Answer from the drawing. Dimensions are ordinates in mm from the lowest x, y and z of the part. A direction names the side the tool comes from. Coordinates: 2 decimals unless noted, no trailing zeros. Order: outer loops, then holes, each group sorted by start corner. A loop starts at its lowest first (then second) coordinate and runs counter-clockwise, first axis right, second up. Notation, with made-up numbers: (11, -3.75) -> (20, -3.75) arc R12 ccw to (20, 17.25) -> close; hole circle Ø2 at (52, -4.5). An arc over 180 degrees is marked (long way). Answer in a Markdown table with one row per item.
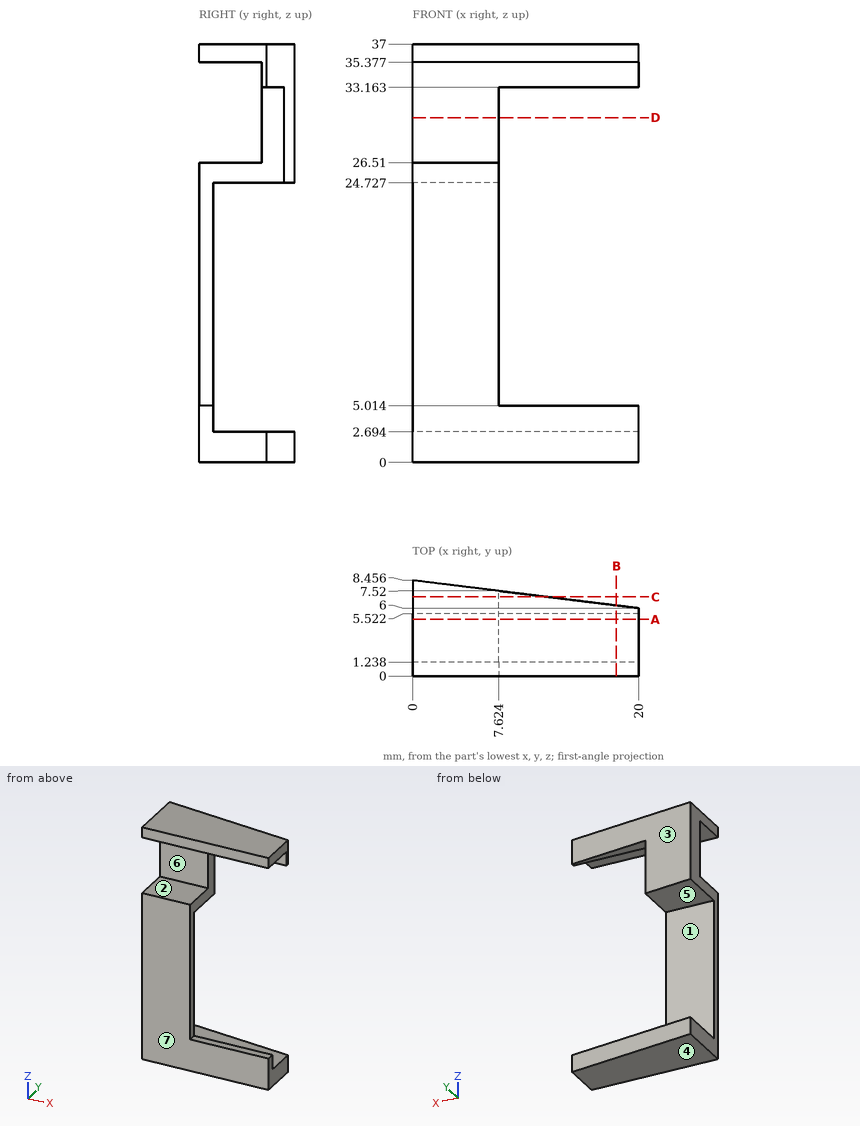
(1) A cutting plane is placed at D-D, the plane z = 30.5. Determine the outline of the cut face in (x, y) (1 decimal).
Check values:
| item | result |
|---|---|
| outline | (0, 5.5) -> (7.6, 5.5) -> (7.6, 7.5) -> (0, 8.5) -> close |
(2) Find the intervals of material crossed by line 1 along Z through (x, y) = (5.25, 6.75) (1 decimal); line 2 along Z through (x, y) = (5.25, 0.75); line 3 along Y through (x, z) = (17, 4), in increasing order. Write a range as from..to.
Check values:
| item | result |
|---|---|
| line 1 | 0..2.7, 24.7..37 |
| line 2 | 0..26.51, 35.38..37 |
| line 3 | 0..1.24 |
(3) Which of the six approach directions +Z, -Z, +X, -X, +Y, -Y give full straight-line access (tool end or side, diameter ignored) to the marked faces 1, 2 and 3?
Check values:
| item | result |
|---|---|
| face 1 | +X, -X, +Y |
| face 2 | +X, -X, -Y |
| face 3 | +Z, -Z, +X, +Y |
(4) For a pull along Z with two mould halves and no side action, classify the marked faces 4, 5, 6 and 7 as released by +Z, released by -Z, zero draft, split by the parting line, or undercut.
Check values:
| item | result |
|---|---|
| face 4 | released by -Z |
| face 5 | undercut |
| face 6 | undercut |
| face 7 | zero draft |
(5) A cutting plane is placed at A-A, the plane y = 5. Determine the outline of the cut face in (x, z) (1 decimal).
Check values:
| item | result |
|---|---|
| outline | (0, 0) -> (20, 0) -> (20, 2.7) -> (0, 2.7) -> close; (0, 24.7) -> (7.6, 24.7) -> (7.6, 26.5) -> (0, 26.5) -> close; (0, 35.4) -> (20, 35.4) -> (20, 37) -> (0, 37) -> close |
(6) A flat-ended cylindrical pin translates along its axis: pin 1 (3 mm diameter, centred on x = 6.5, y = 3.5, fed in from -Z). Find the tip coordinate at first contact, or state that the pin passes through.
Check values:
| item | result |
|---|---|
| pin 1 | z = 0 |
(7) A cutting plane is placed at B-B, the plane x = 18. Determine the outline of the cut face in (y, z) (1 decimal).
Check values:
| item | result |
|---|---|
| outline | (0, 0) -> (6.2, 0) -> (6.2, 2.7) -> (1.2, 2.7) -> (1.2, 5) -> (0, 5) -> close; (0, 35.4) -> (5.5, 35.4) -> (5.5, 33.2) -> (6.2, 33.2) -> (6.2, 37) -> (0, 37) -> close |
(8) A cutting plane is placed at C-C, the plane y = 7. Determine the outline of the cut face in (x, z) (1 decimal).
Check values:
| item | result |
|---|---|
| outline | (0, 0) -> (11.9, 0) -> (11.9, 2.7) -> (0, 2.7) -> close; (0, 24.7) -> (7.6, 24.7) -> (7.6, 33.2) -> (11.9, 33.2) -> (11.9, 37) -> (0, 37) -> close |
